Here's how the part is built. I have some questions about the finished solid (model axes, mm). A direction names the side the tool comes from. Coordinates: 2 decimals unless noted, no trailing zeros. Write each loop counter-clockwise with the first axis right and the second up, starting at its lowest first coordinate (ties: lowest second). Pieces come first, ordered by that corner, then holes. Notation, with made-up numbers: M 58,10.5 L 64,10.5 A21 ccw 64,37.5 Z; hole C 76.25,-6.5 d6. An arc over 180 degrees is marked long. Write each question's results on one line, items separated by ' | '. Start each with the question number.
from build123d import *

# Parameters (mm, degrees)
F1_DEPTH = 4.7625
F2_R     = 2.54


# Not quite as in the source:
# - a length typed as a fraction of an inch, garbled in the dataset ("3 / 203.2 mm" for 3/8 in), is restored


with BuildPart() as f1:
    # F0 (on Top) → F1 (new body)
    with BuildSketch(Plane.XY):
        with BuildLine():
            Line((23.4723398992, 10.7888607308), (23.4723398992, 15.8688607308))
            Line((23.4723398992, 15.8688607308), (-27.3276601008, 15.8688607308))
            Line((-27.3276601008, 15.8688607308), (-27.3276601008, 10.7888607308))
            Line((-27.3276601008, 10.7888607308), (-25.9275856725, 10.7888607308))
            ThreePointArc((-25.9275856725, 10.7888607308), (-24.7369606725, 11.9794857308), (-23.5463356725, 10.7888607308))
            Line((-23.5463356725, 10.7888607308), (-21.4888538531, 10.7888607308))
            ThreePointArc((-21.4888538531, 10.7888607308), (-20.2982288531, 11.9794857308), (-19.1076038531, 10.7888607308))
            Line((-19.1076038531, 10.7888607308), (15.4761500436, 10.7888607308))
            ThreePointArc((15.4761500436, 10.7888607308), (15.7646477316, 12.1575472198), (16.5810500436, 13.2933380835))
            ThreePointArc((16.5810500436, 13.2933380835), (18.8670500436, 14.1797607308), (21.1530500436, 13.2933380835))
            ThreePointArc((21.1530500436, 13.2933380835), (21.9694523555, 12.1575472198), (22.2579500436, 10.7888607308))
            Line((22.2579500436, 10.7888607308), (23.4723398992, 10.7888607308))
        make_face()
        with BuildLine():
            Line((23.4723398992, 5.7088607308), (23.4723398992, 10.7888607308))
            Line((23.4723398992, 10.7888607308), (22.2579500436, 10.7888607308))
            ThreePointArc((22.2579500436, 10.7888607308), (21.9694523555, 9.4201742419), (21.1530500436, 8.2843833782))
            ThreePointArc((21.1530500436, 8.2843833782), (18.8670500436, 7.3979607308), (16.5810500436, 8.2843833782))
            ThreePointArc((16.5810500436, 8.2843833782), (15.7646477316, 9.4201742419), (15.4761500436, 10.7888607308))
            Line((15.4761500436, 10.7888607308), (-19.1076038531, 10.7888607308))
            ThreePointArc((-19.1076038531, 10.7888607308), (-20.2982288531, 9.5982357308), (-21.4888538531, 10.7888607308))
            Line((-21.4888538531, 10.7888607308), (-23.5463356725, 10.7888607308))
            ThreePointArc((-23.5463356725, 10.7888607308), (-24.7369606725, 9.5982357308), (-25.9275856725, 10.7888607308))
            Line((-25.9275856725, 10.7888607308), (-27.3276601008, 10.7888607308))
            Line((-27.3276601008, 10.7888607308), (-27.3276601008, 5.7088607308))
            Line((-27.3276601008, 5.7088607308), (23.4723398992, 5.7088607308))
        make_face()
        with BuildLine():
            Line((16.5810500436, 8.2843833782), (16.5810500436, 10.7888607308))
            Line((16.5810500436, 10.7888607308), (15.4761500436, 10.7888607308))
            ThreePointArc((15.4761500436, 10.7888607308), (15.7646477316, 9.4201742419), (16.5810500436, 8.2843833782))
        make_face()
        with BuildLine():
            Line((15.4761500436, 10.7888607308), (16.5810500436, 10.7888607308))
            Line((16.5810500436, 10.7888607308), (16.5810500436, 13.2933380835))
            ThreePointArc((16.5810500436, 13.2933380835), (15.7646477316, 12.1575472198), (15.4761500436, 10.7888607308))
        make_face()
        with BuildLine():
            Line((21.1530500436, 10.7888607308), (22.2579500436, 10.7888607308))
            ThreePointArc((22.2579500436, 10.7888607308), (21.9694523555, 12.1575472198), (21.1530500436, 13.2933380835))
            Line((21.1530500436, 13.2933380835), (21.1530500436, 10.7888607308))
        make_face()
        with BuildLine():
            ThreePointArc((21.1530500436, 8.2843833782), (21.9694523555, 9.4201742419), (22.2579500436, 10.7888607308))
            Line((22.2579500436, 10.7888607308), (21.1530500436, 10.7888607308))
            Line((21.1530500436, 10.7888607308), (21.1530500436, 8.2843833782))
        make_face()
    extrude(amount=F1_DEPTH)

    # F2
    f2_edges = [f1.edges().sort_by_distance(p)[0] for p in [
        (23.47234, 15.868861, 2.38125),
        (-27.32766, 15.868861, 2.38125),
        (-27.32766, 5.708861, 2.38125),
        (23.47234, 5.708861, 2.38125),
    ]]
    fillet(f2_edges, radius=F2_R)


solid = f1.part
1) Please list where these lines run through material, in increasing order: line 1 (X direction, y = 8.75, z = 1); line 2 (X direction, y = 10, z = 3.9); line 3 (X direction, y = 11, z = 3.65). Write a range as [from, to].
2) I want a section at B-B, the plane z = 1.5. Write out the boundary of the cut face in (x, y).
3) I want a section at A-A, the plane x = 20.5. Write out the boundary of the cut face in (y, z).
4) I want a section at C-C, the plane y = 14.75. Write out the boundary of the cut face in (x, z).
5) For faces 1 (the cylindrical face through (18.9, 7.4, 2.3)), 2 (the cylindrical face through (-26.6, 6.47, 2.41)), which set-ups out of +Z, -Z, +X, -X, +Y, -Y let a thin tool reach every point of the face, with its end or its side?
Output:
1) line 1: x = [-27.33, 16.58], [21.15, 23.47] | line 2: x = [-27.33, -25.63], [-23.85, -21.19], [-19.41, 16.58], [21.15, 23.47] | line 3: x = [-27.33, -25.91], [-23.57, -21.47], [-19.13, 16.58], [21.15, 23.47]
2) outline: M -27.33,8.25 A2.54 ccw -24.79,5.71 L 20.93,5.71 A2.54 ccw 23.47,8.25 L 23.47,13.33 A2.54 ccw 20.93,15.87 L -24.79,15.87 A2.54 ccw -27.33,13.33 Z; hole C -24.74,10.79 d2.38; hole C -20.3,10.79 d2.38; hole M 16.58,8.28 A3.39 ccw 21.15,8.28 L 21.15,13.29 A3.39 ccw 16.58,13.29 Z
3) outline: M 5.71,0 L 7.82,0 L 7.82,4.76 L 5.71,4.76 Z; M 13.76,0 L 15.87,0 L 15.87,4.76 L 13.76,4.76 Z
4) outline: M -26.89,0 L 23.04,0 L 23.04,4.76 L -26.89,4.76 Z
5) face 1: +Z, -Z | face 2: +Z, -Z, -X, -Y
